```python
from build123d import *

# Parameters (mm, degrees)
SKETCH1_W               = 11
SKETCH1_H               = 12
BOSS_EXTRUDE1_DEPTH     = 1.8
SKETCH2_W               = 2.54
SKETCH2_H               = 10.16
BOSS_EXTRUDE2_DEPTH     = 2.54
BOSS_EXTRUDE3_START     = -5.84
SKETCH3_W               = 0.5
SKETCH3_H               = 0.5
BOSS_EXTRUDE3_DEPTH     = 12.34
SKETCH4_W               = 5.5
SKETCH4_H               = 4
BOSS_EXTRUDE4_DEPTH     = 2
CHAMFER1_SIZE           = 0.5
SKETCH5_W               = 0.8
SKETCH5_H               = 7
BOSS_EXTRUDE5_DEPTH     = 0.4
SKETCH6_R               = 0.5
CUT_EXTRUDE1_DEPTH      = 0.1
SKETCH7_R               = 0.25
CUT_EXTRUDE2_DEPTH      = 0.1
SKETCH9_W               = 11
SKETCH9_H               = 12
CUT_EXTRUDE3_DEPTH      = 31
CUT_EXTRUDE4_DEPTH      = 9.381527307
CUT_EXTRUDE4_DEPTH_BACK = 9.381527307
SKETCH10_R              = 0.4


with BuildPart() as part:
    # Sketch1 → Boss-Extrude1 (new body)
    with BuildSketch(Plane(origin=(0, 0, 0), x_dir=(1, 0, 0), z_dir=(0, 1, 0))):
        Rectangle(SKETCH1_W, SKETCH1_H)
    extrude(amount=BOSS_EXTRUDE1_DEPTH)

    # Sketch2 → Boss-Extrude2 (add)
    with BuildSketch(Plane.XZ):
        with Locations((-3.81, 0)):
            Rectangle(SKETCH2_W, SKETCH2_H)
        with Locations((3.81, 0)):
            Rectangle(SKETCH2_W, SKETCH2_H)
    extrude(amount=BOSS_EXTRUDE2_DEPTH)

    # Sketch3 → Boss-Extrude3 (add)
    with BuildSketch(Plane.XZ.offset(2.54).offset(BOSS_EXTRUDE3_START)):
        with Locations((3.81, 1.27)):
            Rectangle(SKETCH3_W, SKETCH3_H)
        with Locations((3.81, 3.81)):
            Rectangle(SKETCH3_W, SKETCH3_H)
        with Locations((3.81, -1.27)):
            Rectangle(SKETCH3_W, SKETCH3_H)
        with Locations((3.81, -3.81)):
            Rectangle(SKETCH3_W, SKETCH3_H)
    boss_extrude3 = extrude(amount=BOSS_EXTRUDE3_DEPTH)

    # Mirror1: Boss-Extrude3 across plane
    add(boss_extrude3.mirror(Plane(origin=(0, 0, 0), x_dir=(0, 0, 1), z_dir=(1, 0, 0))))

    # Sketch4 → Boss-Extrude4 (add)
    with BuildSketch(Plane(origin=(0, 1.8, 0), x_dir=(1, 0, 0), z_dir=(0, 1, 0))):
        Rectangle(SKETCH4_W, SKETCH4_H)
    extrude(amount=BOSS_EXTRUDE4_DEPTH)

    # Chamfer1
    chamfer1_edges = [part.edges().sort_by_distance(p)[0] for p in [
        (0, 3.8, -2),
        (0, 3.8, 2),
    ]]
    chamfer(chamfer1_edges, length=CHAMFER1_SIZE)

    # Sketch5 → Boss-Extrude5 (add)
    with BuildSketch(Plane(origin=(0, 1.8, 0), x_dir=(1, 0, 0), z_dir=(0, 1, 0))):
        with Locations((-0.635, 0)):
            Rectangle(SKETCH5_W, SKETCH5_H)
        with Locations((-1.905, 0)):
            Rectangle(SKETCH5_W, SKETCH5_H)
        with Locations((0.635, 0)):
            Rectangle(SKETCH5_W, SKETCH5_H)
        with Locations((1.905, 0)):
            Rectangle(SKETCH5_W, SKETCH5_H)
    extrude(amount=BOSS_EXTRUDE5_DEPTH)

    # Sketch6 → Cut-Extrude1 (cut)
    with BuildSketch(Plane(origin=(0, 1.8, 0), x_dir=(1, 0, 0), z_dir=(0, 1, 0))):
        with Locations(Location((-3.81, 5.03, 0), (0, 0, 270))):
            Circle(SKETCH6_R)
    extrude(amount=-CUT_EXTRUDE1_DEPTH, mode=Mode.SUBTRACT)

    # Sketch7 → Cut-Extrude2 (cut)
    with BuildSketch(Plane(origin=(0, 3.8, 0), x_dir=(1, 0, 0), z_dir=(0, 1, 0))):
        with Locations(Location((-2.25, -1, 0), (0, 0, 270))):
            Circle(SKETCH7_R)
    extrude(amount=-CUT_EXTRUDE2_DEPTH, mode=Mode.SUBTRACT)

    # Sketch9 → Cut-Extrude3 (cut)
    with BuildSketch(Plane.XZ):
        Rectangle(SKETCH9_W, SKETCH9_H)
    extrude(amount=CUT_EXTRUDE3_DEPTH, mode=Mode.SUBTRACT)

    # Sketch10 → Cut-Extrude4 (cut, two sides: drawn at the far end of the back side and taken through both)
    with BuildSketch(Plane(origin=(0, 1.8, 0), x_dir=(1, 0, 0), z_dir=(0, 1, 0)).offset(-CUT_EXTRUDE4_DEPTH_BACK)):
        with Locations(Location((-3.81, -3.81, 0), (0, 0, 270))):
            Circle(SKETCH10_R)
        with Locations(Location((-3.81, -1.27, 0), (0, 0, 270))):
            Circle(SKETCH10_R)
        with Locations(Location((-3.81, 1.27, 0), (0, 0, 270))):
            Circle(SKETCH10_R)
        with Locations(Location((-3.81, 3.81, 0), (0, 0, 270))):
            Circle(SKETCH10_R)
        with Locations(Location((3.81, -3.81, 0), (0, 0, 90))):
            Circle(SKETCH10_R)
        with Locations(Location((3.81, -1.27, 0), (0, 0, 90))):
            Circle(SKETCH10_R)
        with Locations(Location((3.81, 1.27, 0), (0, 0, 90))):
            Circle(SKETCH10_R)
        with Locations(Location((3.81, 3.81, 0), (0, 0, 90))):
            Circle(SKETCH10_R)
    extrude(amount=CUT_EXTRUDE4_DEPTH + CUT_EXTRUDE4_DEPTH_BACK, mode=Mode.SUBTRACT)


solid = part.part
```
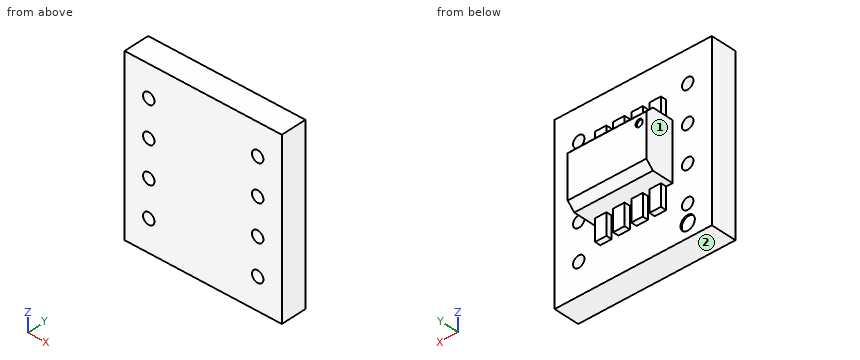
Input: part model. Units: mm. Frame: model coordinates. Face numbers are marked on the shaded views. A direction names the side the tool comes from. Coordinates: 2 decimals unless noted, no trailing zeros. Write each loop counter-clockwise with the first axis right and the second up, starting at its lowest first coordinate (ties: lowest second). Pieces come first, ordered by that corner, then holes. Notation, with made-up numbers: (-24, -2.75) -> (-3, -2.75) arc R9 cw to (-3, 2.25) -> close; hole circle Ø4 at (14.5, 51). An arc over 180 degrees is marked (long way). Write each question's results on one line, items separated by ' | '.
Item 1: Section query B-B on x = -3.81. Return loops of the section in (y, z), plus the area to 3 significant figures.
Conclusion:
outline: (0, -6) -> (1.8, -6) -> (1.8, -5.53) -> (1.7, -5.53) -> (1.7, -4.53) -> (1.8, -4.53) -> (1.8, -4.21) -> (0, -4.21) -> close; (0, -3.41) -> (1.8, -3.41) -> (1.8, -1.67) -> (0, -1.67) -> close; (0, -0.87) -> (1.8, -0.87) -> (1.8, 0.87) -> (0, 0.87) -> close; (0, 1.67) -> (1.8, 1.67) -> (1.8, 3.41) -> (0, 3.41) -> close; (0, 4.21) -> (1.8, 4.21) -> (1.8, 6) -> (0, 6) -> close | area: 15.7 mm^2
Item 2: Section query D-D on z = -5.03. Return loops of the section in (x, y), plus the area to 3 significant figures.
Conclusion:
outline: (-5.5, 0) -> (5.5, 0) -> (5.5, 1.8) -> (-3.31, 1.8) -> (-3.31, 1.7) -> (-4.31, 1.7) -> (-4.31, 1.8) -> (-5.5, 1.8) -> close | area: 19.7 mm^2
Item 3: Section query A-A on z = 3.81. Return loops of the section in (x, y).
Conclusion:
outline: (-5.5, 0) -> (-4.21, 0) -> (-4.21, 1.8) -> (-5.5, 1.8) -> close; (-3.41, 0) -> (3.41, 0) -> (3.41, 1.8) -> (-3.41, 1.8) -> close; (4.21, 0) -> (5.5, 0) -> (5.5, 1.8) -> (4.21, 1.8) -> close
Item 4: Pin query (flat end, axial travel): pin 1 Ø1 at (y, z) = (3, -0.5) entering from -X; pin 2 Ø4 at (x, z) = (1, -5) entering from +Y; pin 3 Ø0.5 at (x, z) = (-4, -5) entering from +Y. Return the tip coordinate at first contact, or that it passes through.
Conclusion:
pin 1: stops at x = -2.75 | pin 2: stops at y = 2.2 | pin 3: stops at y = 1.7
Item 5: Set-up query: the marked faces 1 and 2. Return all of +Z, -Z, +X, -X, +Y, -Y with unobstructed straight access to the full face (end or side cutting, diameter ignored); none if empty.
Conclusion:
face 1: +Z, -Z, -X, +Y | face 2: -Z, +X, -X, +Y, -Y
Item 6: Section query C-C on y = 0.5. Count the separate pieces of the cut face and the enclosed holes in it, plus the area to 3 significant figures.
Conclusion:
separate pieces: 1 | enclosed holes: 8 | area: 128 mm^2
Item 7: Material intervals for probe 1 along X at (y, z) = (0.95, 1.27); probe 2 along Z at (x, y) = (-3.81, 0.75); probe 3 along Z at (x, y) = (-0.25, 3.1), sorted ascending.
Conclusion:
probe 1: x = -5.5 to -4.21, -3.41 to 3.41, 4.21 to 5.5 | probe 2: z = -6 to -4.21, -3.41 to -1.67, -0.87 to 0.87, 1.67 to 3.41, 4.21 to 6 | probe 3: z = -2 to 2
